Solid Edge part; units mm, degrees
sketch "Sketch1" plane through (0, 0, 0) normal (0, 0, 1) x (1, 0, 0)
  line L0 (-40, -50) -> (40, -50)
  line L1 (40, -50) -> (50, -50)
  line L2 (50, -50) -> (50, -40)
  line L3 (50, -40) -> (50, 40)
  line L4 (50, 50) -> (50, 40)
  line L5 (40, 50) -> (50, 50)
  line L6 (40, 50) -> (-40, 50)
  line L7 (-50, 50) -> (-40, 50)
  line L8 (-50, 40) -> (-50, 50)
  line L9 (-50, 40) -> (-50, -40)
  line L10 (-50, -40) -> (-50, -50)
  line L11 (-50, -50) -> (-40, -50)
extrude "Protrusion1" add sketch "Sketch1" against normal blind 5
sketch "Sketch2" plane through (0, 0, 0) normal (0, 0, 1) x (1, 0, 0)
  line L0 (50, 50) -> (40, 50)
  line L1 (40, 46) -> (40, 50)
  line L2 (40, 46) -> (46, 46)
  line L3 (46, 46) -> (46, 40)
  line L4 (46, 40) -> (50, 40)
  line L5 (50, 40) -> (50, 50)
  line L6 (50, -40) -> (50, -50)
  line L7 (50, -50) -> (40, -50)
  line L8 (40, -46) -> (40, -50)
  line L9 (46, -46) -> (40, -46)
  line L10 (46, -40) -> (46, -46)
  line L11 (46, -40) -> (50, -40)
  line L12 (-50, -50) -> (-40, -50)
  line L13 (-40, -46) -> (-40, -50)
  line L14 (-46, -46) -> (-40, -46)
  line L15 (-46, -40) -> (-46, -46)
  line L16 (-50, -40) -> (-46, -40)
  line L17 (-50, -40) -> (-50, -50)
  line L18 (-46, 40) -> (-46, 46)
  line L19 (-46, 46) -> (-40, 46)
  line L20 (-40, 46) -> (-40, 50)
  line L21 (-40, 50) -> (-50, 50)
  line L22 (-50, 50) -> (-50, 40)
  line L23 (-50, 40) -> (-46, 40)
  dimension "D1" = 40
  dimension "D2" = 40
  dimension "D3" = 50
  dimension "D4" = 50
  dimension "D5" = 50
  dimension "D6" = 50
  dimension "D7" = 40
  dimension "D8" = 46
  dimension "D9" = 46
  dimension "D10" = 50
  dimension "D11" = 50
  dimension "D12" = 40
  dimension "D13" = 50
  dimension "D14" = 50
  dimension "D15" = 50
  dimension "D16" = 40
extrude "ExtrudedCutout_1" cut sketch "Sketch2" against normal blind 11.3526
sketch "Sketch3" plane through (0, 0, 0) normal (0, 0, 1) x (1, 0, 0)
  circle A0 centre (-40, -42.86) radius 1.5
  circle A1 centre (-36.13, 42.87) radius 1.5
  circle A2 centre (40, -42.86) radius 1.5
  circle A3 centre (37.53, 42.87) radius 1.5
extrude "Cutout1" cut sketch "Sketch3" against normal blind 5
sketch "Sketch4" plane through (0, 0, 0) normal (0, 0, 1) x (0, 1, 0)
  line L0 (36.87, 44) -> (-36.86, 44)
  line L1 (-36.86, 44) -> (-36.86, 34)
  line L2 (-36.86, 34) -> (-44, 34)
  line L3 (-44, 34) -> (-44, -34)
  line L4 (-44, -34) -> (-36.86, -34)
  line L5 (-36.86, -34) -> (-36.86, -44)
  line L6 (-36.86, -44) -> (36.87, -44)
  line L7 (36.87, -44) -> (36.87, -31.53)
  line L8 (36.87, -31.53) -> (44, -31.53)
  line L9 (44, -31.53) -> (44, 30.13)
  line L10 (44, 30.13) -> (36.87, 30.13)
  line L11 (36.87, 30.13) -> (36.87, 44)
extrude "Cutout2" cut sketch "Sketch4" against normal blind 5
sketch "Sketch5" plane through (0, 0, 0) normal (0, 0, 1) x (1, 0, 0)
  line L0 (-46, 40) -> (-44, 40)
  line L1 (-44, 40) -> (-44, 46)
  line L2 (-44, 46) -> (-46, 46)
  line L3 (-46, 40) -> (-46, 46)
  line L4 (46, 46) -> (44, 46)
  line L5 (44, 46) -> (44, 40)
  line L6 (44, 40) -> (46, 40)
  line L7 (46, 40) -> (46, 46)
  line L8 (-46, -40) -> (-44, -40)
  line L9 (-44, -40) -> (-44, -46)
  line L10 (-44, -46) -> (-46, -46)
  line L11 (-46, -46) -> (-46, -40)
  line L12 (46, -46) -> (44, -46)
  line L13 (44, -46) -> (44, -40)
  line L14 (44, -40) -> (46, -40)
  line L15 (46, -40) -> (46, -46)
extrude "ExtrudedProtrusion_3" add sketch "Sketch5" along normal blind 5
sketch "Sketch6" plane through (-44, -43, 3) normal (1, 0, 0) x (0, 1, 0)
  circle A0 centre (0, -1) radius 1.5
  circle A1 centre (85.9991, -1) radius 1.5
extrude "ExtrudedCutout_14" cut sketch "Sketch6" against normal blind 2
sketch "Sketch7" plane through (44, 43, 2.5) normal (-1, 0, 0) x (0, -1, 0)
  circle A0 centre (0.0009, -0.5) radius 1.5
  circle A1 centre (86, -0.5) radius 1.5
extrude "ExtrudedCutout_15" cut sketch "Sketch7" against normal blind 2
fillet "Round_2" radius 1 8 edges at (45, 40, 5) (45, 46, 5) (-45, 40, 5) (-45, 46, 5) (-45, -46, 5) (-45, -40, 5) (45, -46, 5) (45, -40, 5)
sketch "Sketch8" plane through (0, 0, -5) normal (0, 0, -1) x (0, -1, 0)
  line L0 (-50, -50) -> (50, -50)
  line L1 (50, -50) -> (50, 50)
  line L2 (50, 50) -> (-50, 50)
  line L3 (-50, 50) -> (-50, -50)
  dimension "D1" = 50
  dimension "D2" = 50
extrude "ExtrudedCutout_16" cut sketch "Sketch8" against normal blind 2
sketch "Sketch9" plane through (0, 0, 0) normal (0, 0, 1) x (1, 0, 0)
  line L0 (-36.0661, 36.87) -> (-30.13, 36.87)
  line L1 (-15.0162, 24.5413) -> (-36.0661, 36.87)
  line L2 (-15.0162, 24.5413) -> (15.3161, 6.7761)
  line L3 (-16.3836, -18.795) -> (15.3161, 6.7761)
  line L4 (-16.3836, -18.795) -> (-38.3148, -36.86)
  line L5 (-34, -36.86) -> (-38.3148, -36.86)
  line L6 (-34, -40.7144) -> (-34, -36.86)
  line L7 (-12.6164, -23.465) -> (-34, -40.7144)
  line L8 (-12.6164, -23.465) -> (21.9842, 4.4462)
  line L9 (21.9842, 4.4462) -> (38.2681, 9.0009)
  line L10 (38.2681, 9.0009) -> (44, 10.6041)
  line L11 (44, 10.6041) -> (44, 16.8344)
  line L12 (36.6519, 14.7791) -> (44, 16.8344)
  line L13 (36.6519, 14.7791) -> (20.9991, 10.4009)
  line L14 (-11.9838, 29.7187) -> (20.9991, 10.4009)
  line L15 (-11.9838, 29.7187) -> (-30.13, 40.3467)
  line L16 (-30.13, 40.3467) -> (-30.13, 36.87)
extrude "ExtrudedProtrusion_4" add sketch "Sketch9" against normal blind 3
sketch "Sketch10" plane through (0, 0, 0) normal (0, 0, 1) x (1, 0, 0)
  circle A0 centre (-13.5, 27.13) radius 1.5
  circle A1 centre (37.46, 11.89) radius 1.5
  circle A2 centre (-14.5, -21.13) radius 1.5
extrude "Cutout3" cut sketch "Sketch10" against normal blind 3
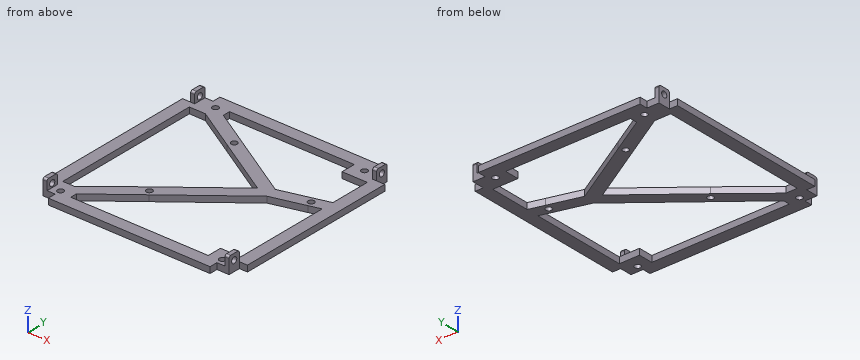
Can you work these out from the model? Positions are in its coordinate system, mm. Give positions to 0.01 mm unless a question says otherwise; leave off trailing zeros. Write each loop counter-clockwise with the first axis right and the second up, starting at its lowest first coordinate (ties: lowest second). Pieces come first, ordered by that corner, then holes. Notation, with made-up numbers: M 67.5,88.5 L 96.5,88.5 A19 ccw 96.5,113.5 Z; hole C 77,16.5 d9. An arc over 180 degrees is marked long. Answer in a Markdown table with one row per item. Add a question column.
Item 1: Imagine slicing it at B-B, the plane y = -42.86. Write out the boundary of the cut face in (x, z).
Item 2: Imagine slicing it at A-A, the plane x = 4. Write out the boundary of the cut face in (y, z).
Item 3: Imagine slicing it at D-D, the plane y = 27.13. Write out the boundary of the cut face in (x, z).
Item 4: Please list where these lines run through material, in increasing order: L1, parallel to Y at x = -36.13, z = -1.6; L2, parallel to X at y = 36.5, z = -1; L3, parallel to Y at x = 16.5, z = -1.5.
Item 5: Imagine slicing it at C-C, the plane y = -9. Write out the boundary of the cut face in (x, z), plus the area to 3 significant figures.
Item 6: For pin 1 Ø4 at (y, z) = (43, 2) entering from +X; pin 2 Ø4 at (x, z) = (-2, 2.5) entering from +Y; pin 3 Ø12 at (x, y) = (4.5, -11.5) entering from +Z; pin 4 Ø4 at (y, z) = (-43, 2) entering from -X, each with a flat end and sliding along its axis, tell me the tip position at first contact or that it passes through.
Evaluation:
| question | item | result |
|---|---|---|
| 1 | outline | M -46,-3 L -41.5,-3 L -41.5,0 L -44,0 L -44,0.51 L -46,0.51 Z; M -46,3.49 L -44,3.49 L -44,5 L -46,5 Z; M -38.5,-3 L -34,-3 L -34,0 L -38.5,0 Z; M 34,-3 L 38.5,-3 L 38.5,0 L 34,0 Z; M 41.5,-3 L 46,-3 L 46,0.51 L 44,0.51 L 44,0 L 41.5,0 Z; M 44,3.49 L 46,3.49 L 46,5 L 44,5 Z |
| 2 | outline | M -50,-3 L -44,-3 L -44,0 L -50,0 Z; M -10.06,-3 L -2.35,-3 L -2.35,0 L -10.06,0 Z; M 13.4,-3 L 20.36,-3 L 20.36,0 L 13.4,0 Z; M 44,-3 L 50,-3 L 50,0 L 44,0 Z |
| 3 | outline | M -50,-3 L -44,-3 L -44,0 L -50,0 Z; M -19.44,-3 L -15,-3 L -15,0 L -19.44,0 Z; M -12,-3 L -7.56,-3 L -7.56,0 L -12,0 Z; M 44,-3 L 50,-3 L 50,0 L 44,0 Z |
| 4 | L1 | y = -50 to -35.06, 36.87 to 41.37, 44.37 to 50 |
| 4 | L2 | x = -50 to -44, -35.43 to -23.56, 44 to 50 |
| 4 | L3 | y = -50 to -44, 0.02 to 13.04, 44 to 50 |
| 5 | outline | M -50,-3 L -44,-3 L -44,0 L -50,0 Z; M -4.24,-3 L 5.32,-3 L 5.32,0 L -4.24,0 Z; M 44,-3 L 50,-3 L 50,0 L 44,0 Z |
| 5 | area | 64.7 mm² |
| 6 | pin 1 | stops at x = 46 |
| 6 | pin 2 | passes through |
| 6 | pin 3 | stops at z = 0 |
| 6 | pin 4 | stops at x = -46 |
